```python
from build123d import *

# Parameters (mm, degrees)
BOSS_EXTRUDE1_DEPTH = 1.9
BOSS_EXTRUDE2_DEPTH = 1
SKETCH3_R           = 3
CUT_EXTRUDE1_DEPTH  = 0.5
SKETCH4_R           = 4.825
SKETCH4_R_2         = 2.775
BOSS_EXTRUDE3_DEPTH = 3.1
SKETCH5_R           = 1.3
CUT_EXTRUDE2_DEPTH  = 3.9
SKETCH6_R           = 0.8
CUT_EXTRUDE4_DEPTH  = 7


with BuildPart() as part:
    # Sketch1 → Boss-Extrude1 (new body)
    with BuildSketch(Plane.XY):
        with BuildLine():
            Line((-5.75, 16), (-5.75, 5.75))
            Line((-5.75, 5.75), (-15, 5.75))
            ThreePointArc((-15, 5.75), (-20.75, 0), (-15, -5.75))
            Line((-15, -5.75), (-5.75, -5.75))
            Line((-5.75, -5.75), (-5.75, -16))
            ThreePointArc((-5.75, -16), (0, -21.75), (5.75, -16))
            Line((5.75, -16), (5.75, -5.75))
            Line((5.75, -5.75), (15, -5.75))
            ThreePointArc((15, -5.75), (20.75, 0), (15, 5.75))
            Line((15, 5.75), (5.75, 5.75))
            Line((5.75, 5.75), (5.75, 16))
            ThreePointArc((5.75, 16), (0, 21.75), (-5.75, 16))
        make_face()
    extrude(amount=BOSS_EXTRUDE1_DEPTH)

    # Sketch2 → Boss-Extrude2 (add)
    with BuildSketch(Plane(origin=(0, 0, 0), x_dir=(-1, 0, 0), z_dir=(0, 0, -1))):
        with BuildLine():
            Line((-5.75, 16), (-5.75, -16))
            ThreePointArc((-5.75, -16), (0, -21.75), (5.75, -16))
            Line((5.75, -16), (5.75, -5.75))
            Line((5.75, -5.75), (5.75, 5.75))
            Line((5.75, 5.75), (5.75, 16))
            ThreePointArc((5.75, 16), (0, 21.75), (-5.75, 16))
        make_face()
    extrude(amount=BOSS_EXTRUDE2_DEPTH)

    # Sketch3 → Cut-Extrude1 (cut)
    with BuildSketch(Plane.XY.offset(1.9)):
        Circle(SKETCH3_R)
    extrude(amount=-CUT_EXTRUDE1_DEPTH, mode=Mode.SUBTRACT)

    # Sketch4 → Boss-Extrude3 (add)
    with BuildSketch(Plane(origin=(0, 0, -1), x_dir=(-1, 0, 0), z_dir=(0, 0, -1))):
        Circle(SKETCH4_R)
        Circle(SKETCH4_R_2, mode=Mode.SUBTRACT)
    extrude(amount=BOSS_EXTRUDE3_DEPTH)

    # Sketch5 → Cut-Extrude2 (cut, through all)
    with BuildSketch(Plane(origin=(0, 0, -1), x_dir=(-1, 0, 0), z_dir=(0, 0, -1))):
        Circle(SKETCH5_R)
    extrude(amount=-CUT_EXTRUDE2_DEPTH, mode=Mode.SUBTRACT)

    # Sketch6 → Cut-Extrude4 (cut, through all)
    with BuildSketch(Plane.XY.offset(1.9)):
        with Locations((-17.95, 0)):
            Circle(SKETCH6_R)
        with Locations((-15.1, 0)):
            Circle(SKETCH6_R)
        with Locations((-12.25, 0)):
            Circle(SKETCH6_R)
        with Locations((0, 18.95)):
            Circle(SKETCH6_R)
        with Locations((0, 16.1)):
            Circle(SKETCH6_R)
        with Locations((0, 13.25)):
            Circle(SKETCH6_R)
        with Locations((12.25, 0)):
            Circle(SKETCH6_R)
        with Locations((15.1, 0)):
            Circle(SKETCH6_R)
        with Locations((17.95, 0)):
            Circle(SKETCH6_R)
        with Locations((0, -10.4)):
            Circle(SKETCH6_R)
        with Locations((0, -13.25)):
            Circle(SKETCH6_R)
        with Locations((0, -16.1)):
            Circle(SKETCH6_R)
        with Locations((0, -18.95)):
            Circle(SKETCH6_R)
        with Locations((0, 10.4)):
            Circle(SKETCH6_R)
    extrude(amount=-CUT_EXTRUDE4_DEPTH, mode=Mode.SUBTRACT)


solid = part.part
```
The listing builds one solid part. Answer for the finished solid, in the listing's coordinates (mm). A direction names the side the tool comes from. Give positions to 0.01 mm unless a question says otherwise; leave off trailing zeros. Loops run counter-clockwise (first coordinate to the right, second up) from the corner with the lowest first, then second, coordinate; pieces in that order, holes last. Notation, with made-up numbers: M 63,23.5 L 113,23.5 A25 ccw 113,36.5 Z; hole C 36,66.5 d2. An arc over 180 degrees is marked long. One line per item, written item: value.
Q1. A cutting plane is placed at D-D on y = 0. Give the number of separate pieces and of enclosed holes in the cut face, then the cut area to 3 significant figures.
Working result:
separate pieces: 8
enclosed holes: 0
area: 75.6 mm^2
Q2. Determine the mould class of faces 4 (the face through (20.75, -0.13, 0.94)), 5 (the face through (13, 1, 0)), 6 (the face through (1.3, 0.7, 1.4)), 7 (the face through (-12.84, 0.54, 0.96)) for opening direction X: +X half, -X half, draft (parallel to the pull), parting line (faces both ways), or undercut.
Working result:
face 4: +X half
face 5: draft
face 6: undercut
face 7: undercut
Q3. For faces 1 (the face through (10, -5.75, 1)), 2 (the face through (-10, -5.75, 1)), 3 (the face through (10, 5.75, 1)), determine the directions among +Z, -Z, +X, -X, +Y, -Y from which every point of the face is accessible in a straight line to the end or side of a thin tool.
Working result:
face 1: +Z, -Z, +X, -Y
face 2: +Z, -Z, -X, -Y
face 3: +Z, -Z, +X, +Y
Q4. A cutting plane is placed at A-A on x = -12.25. Determine the outline of the cut face in (y, z), then the cut area to 3 significant figures.
Working result:
outline: M -5.75,0 L -0.8,0 L -0.8,1.9 L -5.75,1.9 Z; M 0.8,0 L 5.75,0 L 5.75,1.9 L 0.8,1.9 Z
area: 18.8 mm^2
Q5. Find the intervals of material crossed by line 1 (Y direction, x = 15.1, z = 1.25); line 2 (X direction, y = 12, z = 0.3), in increasing order. Write a range as from..to.
Working result:
line 1: y = -5.75..-0.8, 0.8..5.75
line 2: x = -5.75..5.75
Q6. A cutting plane is placed at B-B on y = 13.25. Determine the outline of the cut face in (x, z).
Working result:
outline: M -5.75,-1 L -0.8,-1 L -0.8,1.9 L -5.75,1.9 Z; M 0.8,-1 L 5.75,-1 L 5.75,1.9 L 0.8,1.9 Z
Q7. A cutting plane is placed at C-C on z = -3.15. Determine the outline of the cut face in (x, y) (3 decimals).
Working result:
outline: C 0,0 d9.65; hole C 0,0 d5.55
Q8. Flat-ended cylindrical pins translate along their axes: P1, Ø2, axis at x = -15.1, y = 0, coming from the +Z side; P2, Ø2, axis at x = -17.95, y = 0, coming from the -Z side; P3, Ø1.8, axis at x = 0, y = -18.95, coming from the -Z side; P4, Ø1.8, axis at x = 1.5, y = 0, coming from the +Z side. Find the tip coordinate at first contact, or state that the pin passes through.
Working result:
P1: stops at z = 1.9
P2: stops at z = 0
P3: stops at z = -1
P4: stops at z = 1.4
